Part model, mm, in its own coordinate system. Face numbers are marked on the shaded views. A direction names the side the tool comes from. Coordinates: 2 decimals unless noted, no trailing zeros. Loops run counter-clockwise (first coordinate to the right, second up) from the corner with the lowest first, then second, coordinate; pieces in that order, holes last. Notation, with made-up numbers: (-14, -17.5) -> (32, -17.5) arc R35 cw to (32, 15.5) -> close; hole circle Ø4 at (-38.75, 4.25). An arc over 180 degrees is marked (long way). One line per item, written item: value. Start each with the question number.
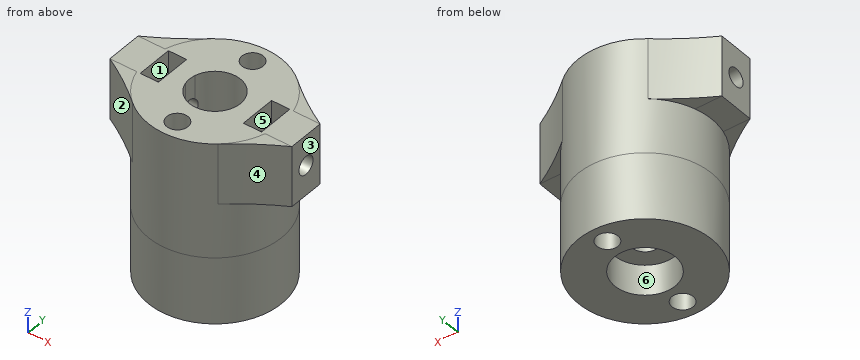
from build123d import *

# Parameters (mm, degrees)
SKETCH1_R               = 11
SKETCH1_R_2             = 1.75
BOSS_EXTRUDE1_DEPTH     = 19
BOSS_EXTRUDE2_START     = 11
SKETCH2_R               = 11
SKETCH2_R_2             = 1.75
BOSS_EXTRUDE2_DEPTH     = 11
CUT_EXTRUDE3_DEPTH      = 20
SKETCH7_R               = 5
CUT_EXTRUDE4_DEPTH      = 5
SKETCH8_R               = 2.2
CUT_EXTRUDE5_DEPTH      = 5
BOSS_EXTRUDE3_DEPTH     = 20
SKETCH11_W              = 3
SKETCH11_H              = 6
CUT_EXTRUDE6_DEPTH      = 10
CUT_EXTRUDE7_DEPTH      = 25.556058316
CUT_EXTRUDE7_DEPTH_BACK = 25.556058316
SKETCH12_R              = 1.5
SKETCH13_W              = 10
SKETCH13_H              = 6
SKETCH13_R              = 1.5
BOSS_EXTRUDE4_DEPTH     = 5
FILLET1_R               = 50


with BuildPart() as part:
    # Sketch1 → Boss-Extrude1 (new body)
    with BuildSketch(Plane.XY):
        Circle(SKETCH1_R)
        with Locations((0, 8)):
            Circle(SKETCH1_R_2, mode=Mode.SUBTRACT)
        with Locations((0, -8)):
            Circle(SKETCH1_R_2, mode=Mode.SUBTRACT)
    extrude(amount=BOSS_EXTRUDE1_DEPTH)

    # Sketch2 → Boss-Extrude2 (add)
    with BuildSketch(Plane(origin=(0, 0, 0), x_dir=(-1, 0, 0), z_dir=(0, 0, -1)).offset(BOSS_EXTRUDE2_START)):
        Circle(SKETCH2_R)
        with Locations((0, 8)):
            Circle(SKETCH2_R_2, mode=Mode.SUBTRACT)
        with Locations((0, -8)):
            Circle(SKETCH2_R_2, mode=Mode.SUBTRACT)
    extrude(amount=-BOSS_EXTRUDE2_DEPTH)

    # Sketch6 → Cut-Extrude3 (cut)
    with BuildSketch(Plane.XY.offset(19)):
        with BuildLine():
            Line((-4.079215611, 1), (-5, 1))
            Line((-5, 1), (-5, -1))
            Line((-5, -1), (-4.079215611, -1))
            ThreePointArc((-4.079215611, -1), (4.2, 0), (-4.079215611, 1))
        make_face()
    extrude(amount=-CUT_EXTRUDE3_DEPTH, mode=Mode.SUBTRACT)

    # Sketch7 → Cut-Extrude4 (cut)
    with BuildSketch(Plane(origin=(0, 0, -11), x_dir=(-1, 0, 0), z_dir=(0, 0, -1))):
        Circle(SKETCH7_R)
    extrude(amount=-CUT_EXTRUDE4_DEPTH, mode=Mode.SUBTRACT)

    # Sketch8 → Cut-Extrude5 (cut)
    with BuildSketch(Plane(origin=(0, 0, -6), x_dir=(-1, 0, 0), z_dir=(0, 0, -1))):
        Circle(SKETCH8_R)
    extrude(amount=-CUT_EXTRUDE5_DEPTH, mode=Mode.SUBTRACT)

    # Sketch9 → Boss-Extrude3 (add)
    with BuildSketch(Plane.XY.offset(19)):
        with BuildLine():
            Line((-5, -1), (-4.079215611, -1))
            ThreePointArc((-4.079215611, -1), (-4.2, 0), (-4.079215611, 1))
            Line((-4.079215611, 1), (-5, 1))
            Line((-5, 1), (-5, -1))
        make_face()
    extrude(amount=-BOSS_EXTRUDE3_DEPTH)

    # Sketch11 → Cut-Extrude6 (cut)
    with BuildSketch(Plane.XY.offset(19)):
        with Locations((-8.5, 0)):
            Rectangle(SKETCH11_W, SKETCH11_H)
        with Locations((8.5, 0)):
            Rectangle(SKETCH11_W, SKETCH11_H)
    extrude(amount=-CUT_EXTRUDE6_DEPTH, mode=Mode.SUBTRACT)

    # Sketch12 → Cut-Extrude7 (cut, two sides: drawn at the far end of the back side and taken through both)
    with BuildSketch(Plane(origin=(0, 0, 0), x_dir=(0, 0, -1), z_dir=(1, 0, 0)).offset(-CUT_EXTRUDE7_DEPTH_BACK)):
        with Locations((-14, 0)):
            Circle(SKETCH12_R)
    extrude(amount=CUT_EXTRUDE7_DEPTH + CUT_EXTRUDE7_DEPTH_BACK, mode=Mode.SUBTRACT)

    # Sketch13 → Boss-Extrude4 (add)
    with BuildSketch(Plane.ZY.offset(-10)):
        with Locations((14, 0)):
            Rectangle(SKETCH13_W, SKETCH13_H)
        with Locations(Location((14, 0, 0), (0, 0, 180))):
            Circle(SKETCH13_R, mode=Mode.SUBTRACT)
    boss_extrude4 = extrude(amount=-BOSS_EXTRUDE4_DEPTH)

    # Mirror1: Boss-Extrude4 across plane
    add(boss_extrude4.mirror(Plane(origin=(0, 0, 0), x_dir=(0, 0, 1), z_dir=(1, 0, 0))))

    # Fillet1
    # the kernel refuses this fillet: 50 mm, written as the material it adds along each edge
    with BuildSketch(Plane(origin=(-10.583005244, -3, 19), x_dir=(0.5439709687724876, -0.8391040371328942, 0), z_dir=(0, 0, -1)), Plane(origin=(10.583005244, 3, 19), x_dir=(-0.5439709687724888, 0.8391040371328933, 0), z_dir=(0, 0, -1))) as fillet1_piece_1:
        with BuildLine():
            CenterArc((21.204232389, 47.782524235), FILLET1_R, 241.826767434, 11.045481443)
            Line((-2.402716916, 3.706318132), (0, 0))
            ThreePointArc((0, 0), (3.239535504, 0.487844668), (6.479071008, 0))
        make_face()
    extrude(amount=10)
    with BuildSketch(Plane(origin=(-10.583005244, 3, 19), x_dir=(0.5439709687724879, 0.839104037132894, 0), z_dir=(0, 0, -1)), Plane(origin=(10.583005244, -3, 19), x_dir=(-0.5439709687724888, -0.8391040371328933, 0), z_dir=(0, 0, -1))) as fillet1_piece_2:
        with BuildLine():
            CenterArc((21.204232389, -47.782524235), FILLET1_R, 107.127751124, 11.045481443)
            Line((-2.402716916, -3.706318132), (0, 0))
            ThreePointArc((0, 0), (3.239535504, -0.487844668), (6.479071008, 0))
        make_face()
    extrude(amount=10)


solid = part.part
1) Tool access for the marked faces 1 and 2: list every direction of +Z, -Z, +X, -X, +Y, -Y with a clear straight run to the whole face (end or side of a thin tool).
2) Pin check, flat tips, straight feed: pin 1 Ø0.9 at (x, z) = (-9, 15.5) entering from +Y; pin 2 Ø4 at (x, y) = (1, 1.5) entering from +Z; pin 3 Ø5 at (x, z) = (9.5, -3) entering from +Y. Stop position of each tip, or through.
3) Slice it at D-D (z = 4.5). Give the cut face in (x, y).
4) Slice it at B-B (x = 0). Give the cut face in (y, z).
5) Pull direction Y, two halves, no side cores. Call the marked faces 3, 4, 5 and 6: +Y half, -Y half, draft (parallel to the pull), parting line (faces both ways), or undercut.
6) Slice it at A-A (z = 14). State how many separate pieces and enclosed holes the cut face has, then the cut area to 3 significant figures.
7) Probe line 1 (Y direction, x = 0, z = -2.55); line 2 (Y direction, x = 0, z = 11); line 3 (X direction, y = 0, z = 8). List the from-to ranges inside material, lowest first. Write a range as from..to.
8) Slice it at C-C (y = 7.5). Give the cut face in (x, z).
Check sheet entries:
1. face 1: +Z
1. face 2: +Z, -Z, -X, -Y
2. pin 1: stops at y = 7.24
2. pin 2: stops at z = -1
2. pin 3: stops at y = 8.49
3. outline: circle Ø22 at (0, 0); hole circle Ø8.4 at (0, 0); hole circle Ø3.5 at (0, -8); hole circle Ø3.5 at (0, 8)
4. outline: (-11, -11) -> (-9.75, -11) -> (-9.75, 19) -> (-11, 19) -> close; (-6.25, -11) -> (-5, -11) -> (-5, -6) -> (-2.2, -6) -> (-2.2, -1) -> (-4.2, -1) -> (-4.2, 19) -> (-6.25, 19) -> close; (2.2, -6) -> (5, -6) -> (5, -11) -> (6.25, -11) -> (6.25, 19) -> (4.2, 19) -> (4.2, -1) -> (2.2, -1) -> close; (9.75, -11) -> (11, -11) -> (11, 19) -> (9.75, 19) -> close
5. face 3: draft
5. face 4: -Y half
5. face 5: undercut
5. face 6: undercut
6. separate pieces: 2
6. enclosed holes: 2
6. area: 305 mm^2
7. line 1: y = -11..-9.75, -6.25..-2.2, 2.2..6.25, 9.75..11
7. line 2: y = -11..-9.75, -6.25..-4.2, 4.2..6.25, 9.75..11
7. line 3: x = -11..-4.2, 4.2..11
8. outline: (-8.21, 9) -> (-8.05, 9) -> (-8.05, -11) -> (-1.68, -11) -> (-1.68, 19) -> (-8.21, 19) -> close; (1.68, -11) -> (8.05, -11) -> (8.05, 9) -> (8.21, 9) -> (8.21, 19) -> (1.68, 19) -> close
